from build123d import *

# Parameters (mm, degrees)
SKETCH2_R           = 4
SKETCH2_W           = 300
SKETCH2_H           = 190
BOSS_EXTRUDE1_DEPTH = 5
SKETCH3_W           = 310
SKETCH3_H           = 200
SKETCH3_W_2         = 300
SKETCH3_H_2         = 190
BOSS_EXTRUDE2_DEPTH = 75
SKETCH4_W           = 310
SKETCH4_H           = 200
BOSS_EXTRUDE3_DEPTH = 5
FILLET2_R           = 15
FILLET3_R           = 15
FILLET4_R           = 15
SKETCH5_R           = 5
CUT_EXTRUDE1_DEPTH  = 5
SKETCH6_W           = 250
SKETCH6_H           = 30
CUT_EXTRUDE2_DEPTH  = 400
SKETCH7_W           = 30
SKETCH7_H           = 145
CUT_EXTRUDE3_DEPTH  = 400
FILLET5_START       = -155
FILLET5_DEPTH       = 5
FILLET5_START_2     = 150
FILLET5_2_DEPTH     = 5
FILLET5_START_3     = -100
FILLET5_3_DEPTH     = 5
FILLET5_START_4     = 95
FILLET5_4_DEPTH     = 5
FILLET5_START_5     = -170
FILLET5_5_DEPTH     = 340
FILLET5_START_6     = -115
FILLET5_6_DEPTH     = 230


with BuildPart() as part:
    # Sketch2 → Boss-Extrude1 (new body)
    with BuildSketch(Plane.XY):
        Polygon((150, -100), (-150, -100), (-150, -115), (-170, -115), (-170, -95), (-155, -95), (-155, 95), (-170, 95), (-170, 115), (-150, 115), (-150, 100), (150, 100), (150, 115), (170, 115), (170, 95), (155, 95), (155, -95), (170, -95), (170, -115), (150, -115), align=None)
        with Locations((-160, 105)):
            Circle(SKETCH2_R, mode=Mode.SUBTRACT)
        with Locations(Location((160, 105, 0), (0, 0, 180))):
            Circle(SKETCH2_R, mode=Mode.SUBTRACT)
        with Locations((160, -105)):
            Circle(SKETCH2_R, mode=Mode.SUBTRACT)
        with Locations(Location((-160, -105, 0), (0, 0, 180))):
            Circle(SKETCH2_R, mode=Mode.SUBTRACT)
        Rectangle(SKETCH2_W, SKETCH2_H, mode=Mode.SUBTRACT)
    extrude(amount=BOSS_EXTRUDE1_DEPTH)

    # Sketch3 → Boss-Extrude2 (add)
    with BuildSketch(Plane.XY.offset(5)):
        Rectangle(SKETCH3_W, SKETCH3_H)
        Rectangle(SKETCH3_W_2, SKETCH3_H_2, mode=Mode.SUBTRACT)
    extrude(amount=BOSS_EXTRUDE2_DEPTH)

    # Sketch4 → Boss-Extrude3 (add)
    with BuildSketch(Plane.XY.offset(80)):
        Rectangle(SKETCH4_W, SKETCH4_H)
    extrude(amount=BOSS_EXTRUDE3_DEPTH)

    # Fillet2
    fillet2_edges = [part.edges().sort_by_distance(p)[0] for p in [
        (-150, 0, 80),
        (0, -95, 80),
        (150, 0, 80),
        (0, 95, 80),
        (150, -95, 40),
        (150, 95, 40),
        (-150, 95, 40),
        (-150, -95, 40),
    ]]
    fillet(fillet2_edges, radius=FILLET2_R)

    # Fillet3
    fillet3_edges = [part.edges().sort_by_distance(p)[0] for p in [
        (-155, -95, 2.5),
        (-150, -100, 2.5),
        (150, -100, 2.5),
        (155, -95, 2.5),
        (155, 95, 2.5),
        (150, 100, 2.5),
        (-155, 95, 2.5),
        (-150, 100, 2.5),
    ]]
    fillet(fillet3_edges, radius=FILLET3_R - 0.0001)  # a hair under: the kernel refuses the full size

    # Fillet4
    fillet4_edges = [part.edges().sort_by_distance(p)[0] for p in [
        (155, -100, 45),
        (155, 100, 45),
        (-155, 0, 85),
        (0, -100, 85),
        (155, 0, 85),
        (0, 100, 85),
        (-155, 100, 45),
        (-155, -100, 45),
    ]]
    fillet(fillet4_edges, radius=FILLET4_R)

    # Sketch5 → Cut-Extrude1 (cut)
    with BuildSketch(Plane(origin=(0, 100, 0), x_dir=(1, 0, 0), z_dir=(0, 1, 0))):
        with Locations(Location((0, -60, 0), (0, 0, 180))):
            Circle(SKETCH5_R)
    extrude(amount=-CUT_EXTRUDE1_DEPTH, mode=Mode.SUBTRACT)

    # Sketch6 → Cut-Extrude2 (cut)
    with BuildSketch(Plane(origin=(0, 100, 0), x_dir=(1, 0, 0), z_dir=(0, 1, 0))):
        Rectangle(SKETCH6_W, SKETCH6_H)
    extrude(amount=-CUT_EXTRUDE2_DEPTH, mode=Mode.SUBTRACT)

    # Sketch7 → Cut-Extrude3 (cut)
    with BuildSketch(Plane(origin=(155, 0, 0), x_dir=(0, 0, -1), z_dir=(1, 0, 0))):
        Rectangle(SKETCH7_W, SKETCH7_H)
    extrude(amount=-CUT_EXTRUDE3_DEPTH, mode=Mode.SUBTRACT)

    # Fillet5: read off the stored shape, not the designer's step
    # Fillet5 outline → Fillet5 (add)
    with BuildSketch(Plane.YZ.offset(FILLET5_START)):
        with BuildLine():
            Line((72.5, 15), (65, 15))
            ThreePointArc((65, 15), (70.303300859, 12.803300859), (72.5, 7.5))
            Line((72.5, 7.5), (72.5, 15))
        make_face()
        with BuildLine():
            Line((-72.5, 15), (-72.5, 7.5))
            ThreePointArc((-72.5, 7.5), (-70.303300859, 12.803300859), (-65, 15))
            Line((-65, 15), (-72.5, 15))
        make_face()
    extrude(amount=FILLET5_DEPTH)

    # Fillet5 2 outline → Fillet5 2 (add)
    with BuildSketch(Plane.YZ.offset(FILLET5_START_2)):
        with BuildLine():
            Line((72.5, 15), (65, 15))
            ThreePointArc((65, 15), (70.303300859, 12.803300859), (72.5, 7.5))
            Line((72.5, 7.5), (72.5, 15))
        make_face()
        with BuildLine():
            Line((-72.5, 15), (-72.5, 7.5))
            ThreePointArc((-72.5, 7.5), (-70.303300859, 12.803300859), (-65, 15))
            Line((-65, 15), (-72.5, 15))
        make_face()
    extrude(amount=FILLET5_2_DEPTH)

    # Fillet5 3 outline → Fillet5 3 (add)
    with BuildSketch(Plane(origin=(0, 0, 0), x_dir=(1, 0, 0), z_dir=(0, 1, 0)).offset(FILLET5_START_3)):
        with BuildLine():
            ThreePointArc((125, -7.5), (122.803300859, -12.803300859), (117.5, -15))
            Line((117.5, -15), (125, -15))
            Line((125, -15), (125, -7.5))
        make_face()
        with BuildLine():
            ThreePointArc((-117.5, -15), (-122.803300859, -12.803300859), (-125, -7.5))
            Line((-125, -7.5), (-125, -15))
            Line((-125, -15), (-117.5, -15))
        make_face()
    extrude(amount=FILLET5_3_DEPTH)

    # Fillet5 4 outline → Fillet5 4 (add)
    with BuildSketch(Plane(origin=(0, 0, 0), x_dir=(1, 0, 0), z_dir=(0, 1, 0)).offset(FILLET5_START_4)):
        with BuildLine():
            ThreePointArc((125, -7.5), (122.803300859, -12.803300859), (117.5, -15))
            Line((117.5, -15), (125, -15))
            Line((125, -15), (125, -7.5))
        make_face()
        with BuildLine():
            ThreePointArc((-117.5, -15), (-122.803300859, -12.803300859), (-125, -7.5))
            Line((-125, -7.5), (-125, -15))
            Line((-125, -15), (-117.5, -15))
        make_face()
    extrude(amount=FILLET5_4_DEPTH)

    # Fillet5 5 outline → Fillet5 5 (cut)
    with BuildSketch(Plane.YZ.offset(FILLET5_START_5)):
        with BuildLine():
            ThreePointArc((80, 0), (74.696699141, 2.196699141), (72.5, 7.5))
            Line((72.5, 7.5), (72.5, 0))
            Line((72.5, 0), (80, 0))
        make_face()
        with BuildLine():
            ThreePointArc((-72.5, 7.5), (-74.696699141, 2.196699141), (-80, 0))
            Line((-80, 0), (-72.5, 0))
            Line((-72.5, 0), (-72.5, 7.5))
        make_face()
    extrude(amount=FILLET5_5_DEPTH, mode=Mode.SUBTRACT)

    # Fillet5 6 outline → Fillet5 6 (cut)
    with BuildSketch(Plane(origin=(0, 0, 0), x_dir=(1, 0, 0), z_dir=(0, 1, 0)).offset(FILLET5_START_6)):
        with BuildLine():
            Line((-125, 0), (-132.5, 0))
            ThreePointArc((-132.5, 0), (-127.196699141, -2.196699141), (-125, -7.5))
            Line((-125, -7.5), (-125, 0))
        make_face()
        with BuildLine():
            Line((125, 0), (125, -7.5))
            ThreePointArc((125, -7.5), (127.196699141, -2.196699141), (132.5, 0))
            Line((132.5, 0), (125, 0))
        make_face()
    extrude(amount=FILLET5_6_DEPTH, mode=Mode.SUBTRACT)


solid = part.part
Build history of the part. All positions in model axes, mm. A direction names the side the tool comes from. Round coordinates to 2 decimals unless told otherwise and drop trailing zeros. Loops run counter-clockwise (first coordinate to the right, second up) from the corner with the lowest first, then second, coordinate; pieces in that order, holes last. Notation, with made-up numbers: (83, 52.25) -> (118, 52.25) arc R13 cw to (118, 63.25) -> close; hole circle Ø2 at (-16, 49.5). An arc over 180 degrees is marked (long way). Answer in a Markdown table with one row per item.
Item 1: Drill centre lines: L1, parallel to Y at x = -109.5, z = 64.5; L2, parallel to X at y = 73, z = 11.5; L3, parallel to Y at x = -94.5, z = 66.5. Where is each one in solid material? Low to high. Write a range as [from, to].
Answers below:
| item | result |
|---|---|
| L1 | y = [-100, -95], [95, 100] |
| L2 | x = [-155, -150], [150, 155] |
| L3 | y = [-100, -94.92], [94.92, 100] |
Item 2: Saw through at A-A (z = 24.5). Write the cut outline in (x, y), and give its area (3 significant figures).
Answers below:
| item | result |
|---|---|
| outline | (-155, -85) arc R15 ccw to (-140, -100) -> (140, -100) arc R15 ccw to (155, -85) -> (155, 85) arc R15 ccw to (140, 100) -> (-140, 100) arc R15 ccw to (-155, 85) -> close; hole (-150, -80) arc R15 ccw to (-135, -95) -> (135, -95) arc R15 ccw to (150, -80) -> (150, 80) arc R15 ccw to (135, 95) -> (-135, 95) arc R15 ccw to (-150, 80) -> close |
| area | 5,000 mm² |
Item 3: Which spindle directions (+Z, -Z, +X, -X, +Y, -Y) get a long thin tool onto all of the face, cutting with end or side? Do faces 5 (the flat face through (-150, -1, 40)), 6 (the flat face through (-156, 102, 5)), 7 (the cylindrical face through (-159.51, -90.72, 2.54)), 8 (the cylindrical face through (159.51, -90.72, 2.54)), 9 (the cylindrical face through (-145.49, -104.28, 2.54)). Say none if no direction does.
Answers below:
| item | result |
|---|---|
| face 5 | -Z |
| face 6 | +Z, -X, +Y |
| face 7 | +Z, -Z, -X |
| face 8 | +Z, -Z, +X |
| face 9 | +Z, -Z, -Y |
Item 4: Saw through at B-B (y = 2). Write the cut outline in (x, z), and give its area (3 significant figures).
Answers below:
| item | result |
|---|---|
| outline | (-155, 15) -> (-150, 15) -> (-150, 65) arc R15 cw to (-135, 80) -> (135, 80) arc R15 cw to (150, 65) -> (150, 15) -> (155, 15) -> (155, 70) arc R15 ccw to (140, 85) -> (-140, 85) arc R15 ccw to (-155, 70) -> close |
| area | 2,200 mm² |
Item 5: Saw through at C-C (x = 160). Write the cut outline in (y, z).
Answers below:
| item | result |
|---|---|
| outline | (-115, 0) -> (-109, 0) -> (-109, 5) -> (-115, 5) -> close; (-101, 0) -> (-91.18, 0) -> (-91.18, 5) -> (-101, 5) -> close; (91.18, 0) -> (101, 0) -> (101, 5) -> (91.18, 5) -> close; (109, 0) -> (115, 0) -> (115, 5) -> (109, 5) -> close |
Item 6: Saw through at D-D (y = 105). Write the cut outline in (x, z).
Answers below:
| item | result |
|---|---|
| outline | (-170, 0) -> (-164, 0) -> (-164, 5) -> (-170, 5) -> close; (-156, 0) -> (-146.18, 0) -> (-146.18, 5) -> (-156, 5) -> close; (146.18, 0) -> (156, 0) -> (156, 5) -> (146.18, 5) -> close; (164, 0) -> (170, 0) -> (170, 5) -> (164, 5) -> close |
Item 7: Pin check, flat tips, straight feed: pin 1 (8 mm diameter, centred on x = -4.5, y = -25.5, fed in from -Z); pin 2 (6 mm diameter, centred on y = 45, z = 15.5, fed in from +X); pin 3 (2 mm diameter, centred on x = 115, z = 64.5, fed in from +Y). Stop position of each tip, or through.
Answers below:
| item | result |
|---|---|
| pin 1 | stops at z = 80 |
| pin 2 | stops at x = 155 |
| pin 3 | stops at y = 100 |
Item 8: Mould opens along Y. For faces 1 (the cylindrical face through (-145.49, -90.72, 32.96)), 2 (the cylindrical face through (-150.72, -95.49, 37.96)), 3 (the cylindrical face through (-150.49, 1.19, 80.72)), 4 (the cylindrical face through (150.49, 95.72, 37.04)) say: +Y half, -Y half, draft (parallel to the pull), parting line (faces both ways), or undercut.
Answers below:
| item | result |
|---|---|
| face 1 | undercut |
| face 2 | -Y half |
| face 3 | draft |
| face 4 | +Y half |
